Read the model definition and answer for the solid it produces. Units are mm, in the model's axes. Round coordinates to 2 decimals unless told otherwise and drop trailing zeros. Order: outer loops, then holes, each group sorted by start corner. A loop starts at its lowest first (then second) coordinate and runs counter-clockwise, first axis right, second up. Notation, with made-up numbers: (60.5, 50) - (77.5, 50) arc R24 ccw to (77.5, 73) - close; hole circle Ø6 at (58.5, 55.5). An arc over 180 degrees is marked (long way). Answer as a JSON object with one key per item and string values. Group by question number.
Q1. A cutting plane is placed at B-B on z = -7.5. Determine the outline of the cut face in (x, y), and give its area (3 significant figures).
Q2. Consider line 1 (Y direction, x = 8.5, z = 57.5); line 2 (Z direction, x = 7, y = 77.5); line 3 (Y direction, x = 4.5, z = -112). Determine where each line is inside the solid, lowest interval first.
Q3. Given pin 1 Ø1.4 at (x, y) = (3.5, 128.5) entering from +Z; pin 2 Ø5 at (y, z) = (125, 142) entering from -X, each flat-ended and moving along its own axis, determine where each tip first touches the part or whether it passes through.
Q4. A cutting plane is placed at A-A on y = 61. Determine the outline of the cut face in (x, z).
Q5. A cutting plane is placed at D-D on x = 8.25. Count the separate pieces of the cut face and the enclosed holes in it, and give its area (3 significant figures).
Q6. A cutting plane is placed at C-C on z = -66.5. Determine the outline of the cut face in (x, y).
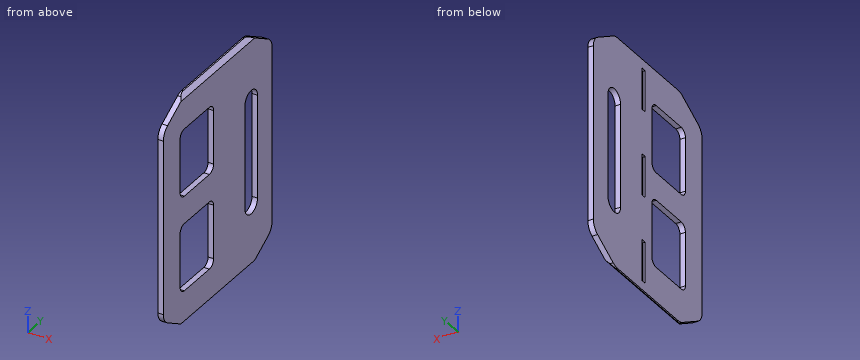
```python
from build123d import *
from OCP.BRepFilletAPI import BRepFilletAPI_MakeChamfer

# Parameters (mm, degrees)
BOSS_EXTRUDE1_DEPTH = 10.16
SKETCH2_W           = 76.2
SKETCH2_H           = 10.16
CUT_EXTRUDE1_DEPTH  = 4.572
CHAMFER1_SIZE       = 38.1
CHAMFER1_SIZE2      = 65.991135768
FILLET1_R           = 25.4


with BuildPart() as part:
    # Sketch1 → Boss-Extrude1 (new body)
    with BuildSketch(Plane(origin=(0, 0, 0), x_dir=(0, 0, -1), z_dir=(1, 0, 0))):
        Polygon((-213.36, 0), (-213.36, 254), (-213.36, 279.4), (213.36, 279.4), (213.36, 254), (213.36, 0), (213.36, -50.8), (-213.36, -50.8), align=None)
        with BuildLine():
            Line((-95.25, 234.95), (95.25, 234.95))
            ThreePointArc((95.25, 234.95), (114.3, 215.9), (95.25, 196.85))
            Line((95.25, 196.85), (-95.25, 196.85))
            ThreePointArc((-95.25, 196.85), (-114.3, 215.9), (-95.25, 234.95))
        make_face(mode=Mode.SUBTRACT)
        with BuildLine():
            Line((38.1, 101.6), (137.16, 101.6))
            ThreePointArc((137.16, 101.6), (146.140256121, 97.880256121), (149.86, 88.9))
            Line((149.86, 88.9), (149.86, 12.7))
            ThreePointArc((149.86, 12.7), (146.140256121, 3.719743879), (137.16, 0))
            Line((137.16, 0), (38.1, 0))
            ThreePointArc((38.1, 0), (29.119743879, 3.719743879), (25.4, 12.7))
            Line((25.4, 12.7), (25.4, 88.9))
            ThreePointArc((25.4, 88.9), (29.119743879, 97.880256121), (38.1, 101.6))
        make_face(mode=Mode.SUBTRACT)
        with BuildLine():
            Line((-38.1, 0), (-137.16, 0))
            ThreePointArc((-137.16, 0), (-146.140256121, 3.719743879), (-149.86, 12.7))
            Line((-149.86, 12.7), (-149.86, 88.9))
            ThreePointArc((-149.86, 88.9), (-146.140256121, 97.880256121), (-137.16, 101.6))
            Line((-137.16, 101.6), (-38.1, 101.6))
            ThreePointArc((-38.1, 101.6), (-29.119743879, 97.880256121), (-25.4, 88.9))
            Line((-25.4, 88.9), (-25.4, 12.7))
            ThreePointArc((-25.4, 12.7), (-29.119743879, 3.719743879), (-38.1, 0))
        make_face(mode=Mode.SUBTRACT)
    extrude(amount=BOSS_EXTRUDE1_DEPTH)

    # Sketch2 → Cut-Extrude1 (cut)
    with BuildSketch(Plane(origin=(0, 0, 0), x_dir=(0, 0, -1), z_dir=(1, 0, 0))):
        with Locations((-158.75, 127)):
            Rectangle(SKETCH2_W, SKETCH2_H)
        with Locations((0, 127)):
            Rectangle(SKETCH2_W, SKETCH2_H)
        with Locations((158.75, 127)):
            Rectangle(SKETCH2_W, SKETCH2_H)
    extrude(amount=CUT_EXTRUDE1_DEPTH, mode=Mode.SUBTRACT)

    # Chamfer1: one chamfer whose edges measure the first distance from different faces: ONE call of the kernel's chamfer builder (chamfer() names one face for all edges)
    chamfer1_edges_1 = [part.edges().sort_by_distance(p)[0] for p in [
        (5.08, 279.4, 213.36),
        (5.08, 279.4, -213.36),
    ]]
    chamfer1_side_1 = [part.faces().sort_by_distance(p)[0] for p in [
        (5.08, 279.4, 0),
    ]]
    chamfer1_edges_2 = [part.edges().sort_by_distance(p)[0] for p in [
        (5.08, -50.8, -213.36),
        (5.08, -50.8, 213.36),
    ]]
    chamfer1_side_2 = [part.faces().sort_by_distance(p)[0] for p in [
        (5.08, -50.8, 0),
    ]]
    chamfer1 = BRepFilletAPI_MakeChamfer(part.part.solid().wrapped)
    for e in chamfer1_edges_1:
        chamfer1.Add(CHAMFER1_SIZE, CHAMFER1_SIZE2, e.wrapped, chamfer1_side_1[0].wrapped)  # the first distance lies on this face
    for e in chamfer1_edges_2:
        chamfer1.Add(CHAMFER1_SIZE, CHAMFER1_SIZE2, e.wrapped, chamfer1_side_2[0].wrapped)  # the first distance lies on this face
    add(Compound.cast(chamfer1.Shape()), mode=Mode.REPLACE)

    # Fillet1
    fillet1_edges = [part.edges().sort_by_distance(p)[0] for p in [
        (5.08, 15.191135768, 213.36),
        (5.08, 213.408864232, 213.36),
        (5.08, 279.4, -175.26),
        (5.08, 279.4, 175.26),
        (5.08, 15.191135768, -213.36),
        (5.08, 213.408864232, -213.36),
        (5.08, -50.8, -175.26),
        (5.08, -50.8, 175.26),
    ]]
    fillet(fillet1_edges, radius=FILLET1_R)

    # Chamfer2
    # the kernel refuses this chamfer: 7.62 mm, written as the material it takes off along each edge
    with BuildSketch(Plane(origin=(10.16, 253.633893228, -213.36), x_dir=(0.02749587661058636, 0, 0.9996219169112968), z_dir=(0, -1, 0))) as chamfer2_piece_1:
        with BuildLine():
            Line((7.838489747, 0), (-0.43088932, 7.826637587))
            Line((-0.43088932, 7.826637587), (-0.5832317, 7.822447215))
            ThreePointArc((-0.5832317, 7.822447215), (-0.26006471, 3.912091462), (-0.15234238, -0.004190372))
            Line((-0.15234238, -0.004190372), (0.004190372, -0.15234238))
            ThreePointArc((0.004190372, -0.15234238), (3.920472205, -0.04462005), (7.842680119, -0.15234238))
            Line((7.842680119, -0.15234238), (7.838489747, 0))
        make_face()
    extrude(amount=278.667786456, mode=Mode.SUBTRACT)
    with BuildSketch(Plane(origin=(10.16, -25.033893228, 213.36), x_dir=(-0.9996219169112968, 0, 0.027495876610586382), z_dir=(0, 1, 0))) as chamfer2_piece_2:
        with BuildLine():
            Line((7.838489747, 0), (-0.43088932, -7.826637587))
            Line((-0.43088932, -7.826637587), (-0.5832317, -7.822447215))
            ThreePointArc((-0.5832317, -7.822447215), (-0.26006471, -3.912091462), (-0.15234238, 0.004190372))
            Line((-0.15234238, 0.004190372), (0.004190372, 0.15234238))
            ThreePointArc((0.004190372, 0.15234238), (3.920472205, 0.04462005), (7.842680119, 0.15234238))
            Line((7.842680119, 0.15234238), (7.838489747, 0))
        make_face()
    extrude(amount=278.667786456, mode=Mode.SUBTRACT)


solid = part.part
```
Result set:
{
 "1": {"outline": "(0, -50.8) - (10.16, -50.8) - (10.16, 196.85) - (0, 196.85) - (0, 132.08) - (4.57, 132.08) - (4.57, 121.92) - (0, 121.92) - close; (0, 234.95) - (10.16, 234.95) - (10.16, 279.4) - (0, 279.4) - close", "area": "2,920 mm²"},
 "2": {"line 1": "y = -50.8 to 0, 101.6 to 196.85, 234.95 to 279.4", "line 2": "z = -208.9 to -149.86, -25.4 to 25.4, 149.86 to 208.9", "line 3": "y = -50.8 to 0, 101.6 to 206.83, 224.97 to 279.4"},
 "3": {"pin 1": "stops at z = 213.1", "pin 2": "stops at x = 4.57"},
 "4": {"outline": "(0, -213.36) - (2.54, -213.36) - (10.16, -205.74) - (10.16, -149.86) - (0, -149.86) - close; (0, -25.4) - (10.16, -25.4) - (10.16, 25.4) - (0, 25.4) - close; (0, 149.86) - (10.16, 149.86) - (10.16, 205.74) - (2.54, 213.36) - (0, 213.36) - close"},
 "5": {"separate pieces": "1", "enclosed holes": "3", "area": "99,900 mm²"},
 "6": {"outline": "(0, -50.8) - (10.16, -50.8) - (10.16, 0) - (0, 0) - close; (0, 101.6) - (10.16, 101.6) - (10.16, 196.85) - (0, 196.85) - close; (0, 234.95) - (10.16, 234.95) - (10.16, 279.4) - (0, 279.4) - close"}
}
